from build123d import *

# Parameters (mm, degrees)
F0_R     = 2.875
F1_DEPTH = 12
F0_R_2   = 4.425
F2_DEPTH = 2.2
F3_SIZE  = 1
F4_R     = 0.5


with BuildPart() as f1:
    # F0 (on Top) → F1 (new body)
    with BuildSketch(Plane.XY):
        Circle(F0_R)
    extrude(amount=F1_DEPTH)

    # F0 (on Top) → F2 (join)
    with BuildSketch(Plane.XY):
        Circle(F0_R_2)
        Circle(F0_R, mode=Mode.SUBTRACT)
    extrude(amount=F2_DEPTH)

    # F3
    f3_edges = [f1.edges().sort_by_distance(p)[0] for p in [
        (-2.875, 0, 12),
    ]]
    chamfer(f3_edges, length=F3_SIZE)

    # F4
    f4_edges = [f1.edges().sort_by_distance(p)[0] for p in [
        (-4.425, 0, 2.2),
        (-2.875, 0, 2.2),
    ]]
    fillet(f4_edges, radius=F4_R)


solid = f1.part
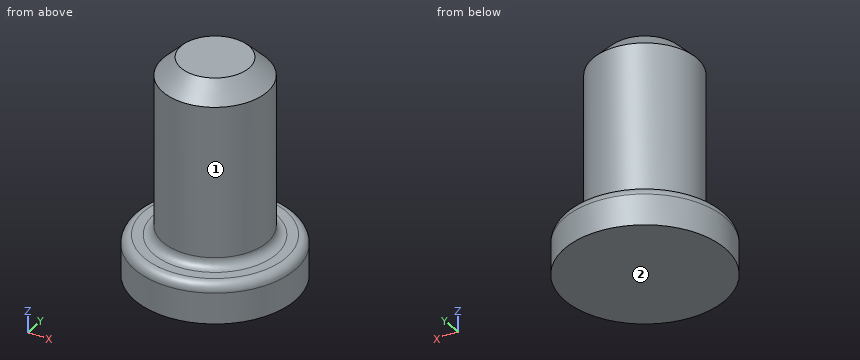
Geometry: final body of the model. Coordinates: model frame, mm. Face numbers are marked on the shaded views. A direction names the side the tool comes from. Coordinates: 2 decimals unless noted, no trailing zeros. Loops run counter-clockwise (first coordinate to the right, second up) from the corner with the lowest first, then second, coordinate; pieces in that order, holes last. Notation, with made-up numbers: M 32.5,62 L 60.5,62 A6 ccw 60.5,66 Z; hole C -33.5,-2 d1. An arc over 180 degrees is marked long. One line per item, written item: value. Start each with the question number.
1) Cut plane C-C (z = 5). Return loops of the section in (x, y) (3 decimals), then the cut area to 3 significant figures.
2) Material intervals for L1, parallel to Z at x = -0.5, y = 3.5; L2, parallel to Y at x = -0.25, z = 0.5; L3, parallel to X at y = -0.75, z = 3, sorted ascending. Write a range as from..to.
3) Pin query (flat end, axial travel): P1, Ø1, axis at x = -2, z = 4, coming from the -Y side; P2, Ø3, axis at y = 1.5, z = 2.5, coming from the -X side; P3, Ø5, axis at x = -2.5, y = -1.5, coming from the -Z side; P4, Ø2, axis at x = -2, z = 5.5, coming from the -Y side. Return the tip coordinate at first contact, or that it passes through.
4) Reachability of the marked faces 1 and 2 from +Z, -Z, +X, -X, +Y, -Y: full face, straight path, thin tool, end or side. Return the list, or none.
5) Cut plane A-A (y = 0). Return loops of the section in (x, z) (3 decimals).
6) Cut plane D-D (z = 2.5). Return loops of the section in (x, y), then the cut area to 3 significant figures.
Evaluation:
1. outline: C 0,0 d5.75
1. area: 26.0 mm^2
2. L1: 0..2.2
2. L2: -4.42..4.42
2. L3: -2.78..2.78
3. P1: y = -2.45
3. P2: x = -4.42
3. P3: z = 0
3. P4: y = -2.7
4. face 1: +Z
4. face 2: -Z, +X, -X, +Y, -Y
5. outline: M -4.425,0 L 4.425,0 L 4.425,1.7 A0.5 ccw 3.925,2.2 L 3.375,2.2 A0.5 cw 2.875,2.7 L 2.875,11 L 1.875,12 L -1.875,12 L -2.875,11 L -2.875,2.7 A0.5 cw -3.375,2.2 L -3.925,2.2 A0.5 ccw -4.425,1.7 Z
6. outline: C 0,0 d5.83
6. area: 26.7 mm^2
